Part print with two shaded views. Sizes in mm from the minimum x, y, z corner. A direction names the side the tool comes from. Round coordinates to 2 decimals unless told otherwise and drop trailing zeros. Order: outer loops, then holes, each group sorted by start corner. A loop starts at its lowest first (then second) coordinate and runs counter-clockwise, first axis right, second up. Notation, with made-up numbers: (36, 15.5) - (72, 15.5) arc R23 ccw to (72, 23.5) - close; hole circle Ø2 at (-6, -3.75). An arc over 180 degrees is marked (long way). Use one line per item in the form item = value.
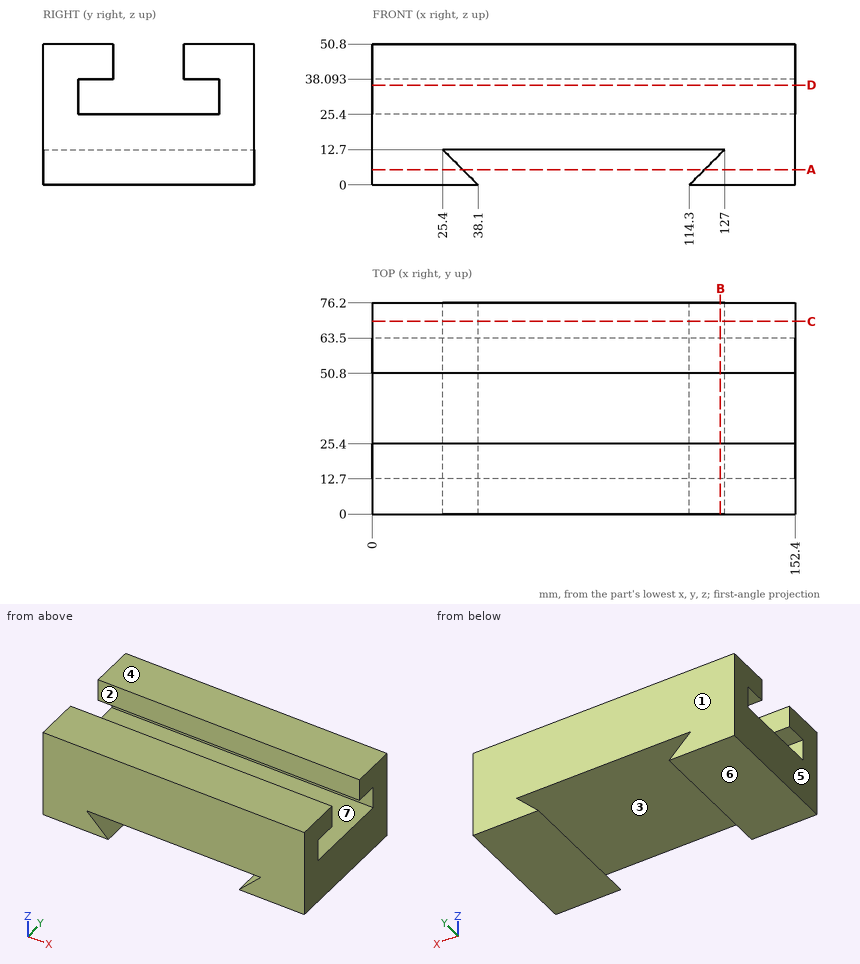
(1) Tool access for the marked faces 1, 2 and 3: list every direction of +Z, -Z, +X, -X, +Y, -Y with a clear straight run to the whole face (end or side of a thin tool).
Report:
face_1 = +Z, -Z, +X, -X, +Y
face_2 = +Z, +X, -X
face_3 = +Y, -Y
(2) Slice it at B-B on x = 125.5. Give the cut face in (y, z).
Report:
outline = (0, 0) - (76.2, 0) - (76.2, 11.2) - (0, 11.2) - close; (0, 12.7) - (76.2, 12.7) - (76.2, 50.8) - (50.8, 50.8) - (50.8, 38.09) - (63.5, 38.09) - (63.5, 25.4) - (12.7, 25.4) - (12.7, 38.09) - (25.4, 38.09) - (25.4, 50.8) - (0, 50.8) - close
(3) Slice it at D-D on z = 36. Give the cut face in (x, y), then the cut area to 3 significant figures.
Report:
outline = (0, 0) - (152.4, 0) - (152.4, 12.7) - (0, 12.7) - close; (0, 63.5) - (152.4, 63.5) - (152.4, 76.2) - (0, 76.2) - close
area = 3,870 mm2
(4) Pin check, flat tips, straight feed: pin 1 (1.5 mm diameter, centred on x = 116, y = 49, fed in from +Z); pin 2 (14 mm diameter, centred on x = 68.5, y = 55.5, fed in from -Z). Stop position of each tip, or through.
Report:
pin_1 = 25.4
pin_2 = 12.7
(5) Slice it at C-C on y = 69.5. Give the cut face in (x, z), then the cut area to 3 significant figures.
Report:
outline = (0, 0) - (38.1, 0) - (25.4, 12.7) - (127, 12.7) - (114.3, 0) - (152.4, 0) - (152.4, 50.8) - (0, 50.8) - close
area = 6,610 mm2
(6) Pull direction Z, two halves, no side cores. Call the marked faces 4, 5, 6 and 7: released by +Z, released by -Z, zero draft, split by the parting line, or undercut.
Report:
face_4 = released by +Z
face_5 = zero draft
face_6 = released by -Z
face_7 = undercut
(7) Slice it at A-A on z = 5.5. Give the cut face in (x, y).
Report:
outline = (0, 0) - (32.6, 0) - (32.6, 76.2) - (0, 76.2) - close; (119.8, 0) - (152.4, 0) - (152.4, 76.2) - (119.8, 76.2) - close
(8) Probe probe 1 along Z at (x, y) = (74, 17.5); probe 2 along Y at (x, z) = (87.5, 41); probe 3 along Z at (x, y) = (128, 59). List the from-to ranges inside material, lowest first. Write a range as [from, to].
Report:
probe_1 = [12.7, 25.4], [38.09, 50.8]
probe_2 = [0, 25.4], [50.8, 76.2]
probe_3 = [0, 25.4], [38.09, 50.8]
